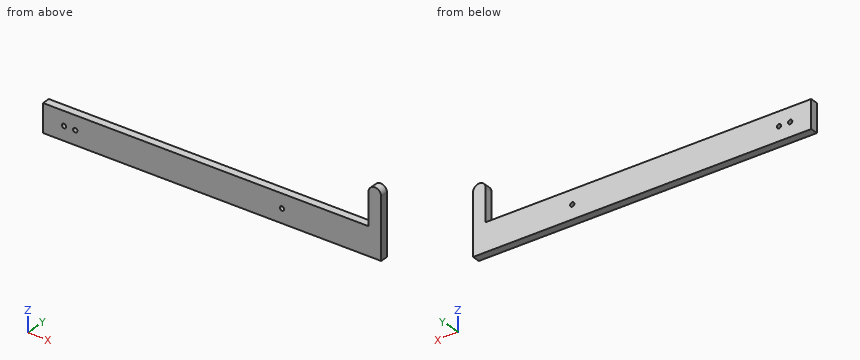
```python
from build123d import *

# Parameters (mm, degrees)
SKETCH1_W           = 241.3
SKETCH1_H           = 20
BOSS_EXTRUDE1_DEPTH = 5.588
CUT_EXTRUDE1_REACH  = 169.751
SKETCH2_R           = 1.525
SKETCH3_W           = 9
SKETCH3_H           = 23
BOSS_EXTRUDE2_DEPTH = 5.588
BOSS_EXTRUDE3_DEPTH = 5.588


with BuildPart() as part:
    # Sketch1 → Boss-Extrude1 (new body)
    with BuildSketch(Plane(origin=(0, 0, 0), x_dir=(1, 0, 0), z_dir=(0, 1, 0))):
        with Locations((-46.608825085, 1.565543133)):
            Rectangle(SKETCH1_W, SKETCH1_H)
    extrude(amount=BOSS_EXTRUDE1_DEPTH)

    # Sketch2 → Cut-Extrude1 (cut, up to next)
    with BuildSketch(Plane(origin=(0, 5.588, 0), x_dir=(1, 0, 0), z_dir=(0, 1, 0)), mode=Mode.PRIVATE) as cut_extrude1_sk1:
        with Locations(Location((3.241174915, 1.565543133, 0), (0, 0, 270))):
            Circle(SKETCH2_R)
    cut_extrude1_tool1 = extrude(cut_extrude1_sk1.sketch, amount=-CUT_EXTRUDE1_REACH, mode=Mode.PRIVATE) & part.part
    # Sketch2 → Cut-Extrude1 (cut, up to next)
    with BuildSketch(Plane(origin=(0, 5.588, 0), x_dir=(1, 0, 0), z_dir=(0, 1, 0)), mode=Mode.PRIVATE) as cut_extrude1_sk2:
        with Locations(Location((-152.258825085, 1.565543133, 0), (0, 0, 270))):
            Circle(SKETCH2_R)
    cut_extrude1_tool2 = extrude(cut_extrude1_sk2.sketch, amount=-CUT_EXTRUDE1_REACH, mode=Mode.PRIVATE) & part.part
    # Sketch2 → Cut-Extrude1 (cut, up to next)
    with BuildSketch(Plane(origin=(0, 5.588, 0), x_dir=(1, 0, 0), z_dir=(0, 1, 0)), mode=Mode.PRIVATE) as cut_extrude1_sk3:
        with Locations(Location((-144.258825085, 1.565543133, 0), (0, 0, 270))):
            Circle(SKETCH2_R)
    cut_extrude1_tool3 = extrude(cut_extrude1_sk3.sketch, amount=-CUT_EXTRUDE1_REACH, mode=Mode.PRIVATE) & part.part
    add(cut_extrude1_tool1.solids().sort_by_distance((3.241175, 5.588, -1.565543))[0], mode=Mode.SUBTRACT)
    add(cut_extrude1_tool2.solids().sort_by_distance((-152.258825, 5.588, -1.565543))[0], mode=Mode.SUBTRACT)
    add(cut_extrude1_tool3.solids().sort_by_distance((-144.258825, 5.588, -1.565543))[0], mode=Mode.SUBTRACT)

    # Sketch3 → Boss-Extrude2 (add)
    with BuildSketch(Plane(origin=(0, 5.588, 0), x_dir=(1, 0, 0), z_dir=(0, 1, 0))):
        with Locations((69.541174915, -19.934456867)):
            Rectangle(SKETCH3_W, SKETCH3_H)
    extrude(amount=-BOSS_EXTRUDE2_DEPTH)

    # Sketch4 → Boss-Extrude3 (add)
    with BuildSketch(Plane(origin=(0, 5.588, 0), x_dir=(1, 0, 0), z_dir=(0, 1, 0))):
        with BuildLine():
            Line((65.041174915, -31.434456867), (74.041174915, -31.434456867))
            ThreePointArc((74.041174915, -31.434456867), (69.541174915, -35.934456867), (65.041174915, -31.434456867))
        make_face()
    extrude(amount=-BOSS_EXTRUDE3_DEPTH)


solid = part.part
```
CAD build for the part. Positions are in the model's coordinates, mm. Coordinates: 2 decimals unless noted, no trailing zeros. Write each loop counter-clockwise with the first axis right and the second up, starting at its lowest first coordinate (ties: lowest second). Pieces come first, ordered by that corner, then holes. Notation, with made-up numbers: (32, -39.75) -> (75, -39.75) arc R9 cw to (75, -30.75) -> close; hole circle Ø3 at (82.5, -18). An arc over 180 degrees is marked (long way). Return JSON: item names as keys, results as strings. Group by question number.
Q1. Drill centre lines: line 1 (X direction, y = 1.45, z = -1.5); line 2 (X direction, y = 4.6, z = -2.5); line 3 (X direction, y = 2.1, z = 32). Where is each one in solid material? Low to high.
Q2. Cut at C-C, the plane x = 57. Give the cut face in (y, z).
Q3. Cut at A-A, the plane y = 2.3. Give the cut face in (x, z) (3 decimals), then the cut area to 3 significant figures.
Q4. Cut at B-B, the plane z = 29. Give the cut face in (x, y).
Q5. Flat gauge pins, fed straight in: pin 1 (3.5 mm diameter, centred on x = 3.24, z = -1.57, fed in from +Y); pin 2 (2.5 mm diameter, centred on x = -152.26, z = -1.57, fed in from +Y). Where does each tip first touch, or does it go through?
Returned:
{
 "1": {"line 1": "x = -167.26 to -153.78, -150.74 to -145.78, -142.74 to 1.72, 4.76 to 74.04", "line 2": "x = -167.26 to -153.46, -151.05 to -145.46, -143.05 to 2.04, 4.45 to 74.04", "line 3": "x = 65.08 to 74.01"},
 "2": {"outline": "(0, -11.57) -> (5.59, -11.57) -> (5.59, 8.43) -> (0, 8.43) -> close"},
 "3": {"outline": "(-167.259, -11.566) -> (74.041, -11.566) -> (74.041, 31.434) arc R4.5 ccw to (65.041, 31.434) -> (65.041, 8.434) -> (-167.259, 8.434) -> close; hole circle Ø3.05 at (-152.259, -1.566); hole circle Ø3.05 at (-144.259, -1.566); hole circle Ø3.05 at (3.241, -1.566)", "area": "5,040 mm2"},
 "4": {"outline": "(65.04, 0) -> (74.04, 0) -> (74.04, 5.59) -> (65.04, 5.59) -> close"},
 "5": {"pin 1": "stops at y = 5.59", "pin 2": "passes through"}
}
